```python
from build123d import *

# Parameters (mm, degrees)
F0_W     = 33.5
F0_H     = 21
F0_H_2   = 2
F0_H_3   = 15
F0_R     = 0.6
F3_DEPTH = 1.5
F1_W     = 33.5
F1_H     = 20
F4_DEPTH = 1.5
F5_DEPTH = 1
F8_DEPTH = 1
F9_DEPTH = 3


with BuildPart() as f3:
    # F0 (on Front) → F3 (new body)
    with BuildSketch(Plane.XZ):
        with Locations((-16.75, 27.5)):
            Rectangle(F0_W, F0_H)
        with Locations((-16.75, 16)):
            Rectangle(F0_W, F0_H_2)
        with Locations((-16.75, 7.5)):
            Rectangle(F0_W, F0_H_3)
        with BuildLine():
            Line((-35, 15), (-33.5, 15))
            Line((-33.5, 15), (-33.5, 17))
            Line((-33.5, 17), (-35, 17))
            ThreePointArc((-35, 17), (-36, 16), (-35, 15))
        make_face()
        with Locations((-35, 16)):
            Circle(F0_R, mode=Mode.SUBTRACT)
        with BuildLine():
            Line((0, 17), (0, 15))
            Line((0, 15), (1.5, 15))
            ThreePointArc((1.5, 15), (2.5, 16), (1.5, 17))
            Line((1.5, 17), (0, 17))
        make_face()
        with Locations((1.5, 16)):
            Circle(F0_R, mode=Mode.SUBTRACT)
    extrude(amount=F3_DEPTH)

    # F1 (on Top) → F4 (join)
    with BuildSketch(Plane.XY):
        with Locations((-16.75, -10)):
            Rectangle(F1_W, F1_H)
    extrude(amount=F4_DEPTH)

    # F2 (on Right) → F5 (join)
    with BuildSketch(Plane.YZ):
        Polygon((-9.024499878, 0), (-8, 0), (0, 10), (0, 11.2806248475), align=None)
    extrude(amount=-F5_DEPTH)

    # F7 (on offset) → F8 (join)
    with BuildSketch(Plane.YZ.offset(-32.5)):
        Polygon((-8.8, 0), (-8, 0), (0, 10), (0, 10.8), align=None)
    extrude(amount=-F8_DEPTH)

    # F0 (on Front) → F9 (join)
    with BuildSketch(Plane.XZ):
        with BuildLine():
            Line((-35, 15), (-33.5, 15))
            Line((-33.5, 15), (-33.5, 17))
            Line((-33.5, 17), (-35, 17))
            ThreePointArc((-35, 17), (-36, 16), (-35, 15))
        make_face()
        with Locations((-35, 16)):
            Circle(F0_R, mode=Mode.SUBTRACT)
        with BuildLine():
            Line((0, 17), (0, 15))
            Line((0, 15), (1.5, 15))
            ThreePointArc((1.5, 15), (2.5, 16), (1.5, 17))
            Line((1.5, 17), (0, 17))
        make_face()
        with Locations((1.5, 16)):
            Circle(F0_R, mode=Mode.SUBTRACT)
    extrude(amount=-F9_DEPTH)


solid = f3.part
```
Input: part model. Units: mm. Frame: model coordinates. A direction names the side the tool comes from. Round coordinates to 2 decimals unless told otherwise and drop trailing zeros. Loops run counter-clockwise (first coordinate to the right, second up) from the corner with the lowest first, then second, coordinate; pieces in that order, holes last. Notation, with made-up numbers: M 66.25,27 L 83.25,27 A16 ccw 83.25,32 Z; hole C 19.25,15 d11. An arc over 180 degrees is marked long. Answer in a Markdown table with one row per item. Add a question column.
1. Set-up query: faces 1 (the face through (-33.5, -1, 28)), 2 (the face through (-33, -4, 5)), 3 (the face through (-32.5, -4.3, 5)), 4 (the face through (-34, 1, 15)), 5 (the face through (-32.99, -4.5, 5.28)). Return all of +Z, -Z, +X, -X, +Y, -Y with unobstructed straight access to the full face (end or side cutting, diameter ignored); none if empty.
2. Section C-C (y = -5.5). Output: boundary loops of the cut face in (x, z) (3 decimals).
3. Ray query, probe 1 along Z at (x, y) = (-35, 1.95); probe 2 along X at (y, z) = (-6, 3); probe 3 along Y at (x, z) = (-24.5, 33.5). Return the intervals inside material, ascending.
4. Mould query, pull axis X, two halves, no side actions, for faces 6 (the face through (-1, -4.4, 4.9)), 7 (the face through (0, -1, 27)), 8 (the face through (-34, 1, 17)). Classes: released by +X, released by -X, zero draft, split by the parting line, or undercut.
5. Section A-A (z = 16). Output: boundary loops of the cut face in (x, y), and give its area (4 significant figures).
6. Contact query for flat-ended pins moving along their axis: pin 1 (12 mm diameter, centred on x = -11.5, y = -8, fed in from +Z); pin 2 (0.8 mm diameter, centred on x = -34, y = 1, fed in from +Z); pin 3 (3 mm diameter, centred on x = -22.5, z = 12.5, fed in from +Y); pin 4 (6 mm diameter, centred on x = -29.5, y = -10.5, fed in from -Z). Output: stop coordinate, or through.
7. Section D-D (x = -13.5). Output: boundary loops of the cut face in (y, z), and give its area (4 significant figures).
8. Section B-B (y = -0.75). Output: boundary loops of the cut face in (x, z), and give its area (3 significant figures).
Values follow:
| question | item | result |
|---|---|---|
| 1 | face 1 | +Z, -X, +Y, -Y |
| 1 | face 2 | +X, -X |
| 1 | face 3 | +Z, -Y |
| 1 | face 4 | -Z, -X, +Y, -Y |
| 1 | face 5 | +Z, -X, -Y |
| 2 | outline | M -33.5,0 L 0,0 L 0,1.5 L -33.5,1.5 Z; M -33.5,3.125 L -32.5,3.125 L -32.5,4.05 L -33.5,4.05 Z; M -1,3.125 L 0,3.125 L 0,4.406 L -1,4.406 Z |
| 3 | probe 1 | 15 to 15.4, 16.6 to 17 |
| 3 | probe 2 | -33.5 to -32.5, -1 to 0 |
| 3 | probe 3 | -1.5 to 0 |
| 4 | face 6 | undercut |
| 4 | face 7 | released by +X |
| 4 | face 8 | zero draft |
| 5 | outline | M -36,-1.5 L -35.6,-1.5 L -35.6,3 L -36,3 Z; M -34.4,-1.5 L 0.9,-1.5 L 0.9,3 L 0,3 L 0,0 L -33.5,0 L -33.5,3 L -34.4,3 Z; M 2.1,-1.5 L 2.5,-1.5 L 2.5,3 L 2.1,3 Z |
| 5 | area | 61.95 mm^2 |
| 6 | pin 1 | z = 1.5 |
| 6 | pin 2 | z = 17 |
| 6 | pin 3 | y = 0 |
| 6 | pin 4 | z = 0 |
| 7 | outline | M -20,0 L 0,0 L 0,38 L -1.5,38 L -1.5,1.5 L -20,1.5 Z |
| 7 | area | 84.75 mm^2 |
| 8 | outline | M -35,15 L -33.5,15 L -33.5,0 L 0,0 L 0,15 L 1.5,15 A1 ccw 1.5,17 L 0,17 L 0,38 L -33.5,38 L -33.5,17 L -35,17 A1 ccw Z; hole C -35,16 d1.2; hole C 1.5,16 d1.2 |
| 8 | area | 1,280 mm^2 |
